```python
from build123d import *

# Parameters (mm, degrees)
F0_W     = 25
F0_H     = 25
F1_DEPTH = 17.5
F2_W     = 25
F2_H     = 25
F3_DEPTH = 15


with BuildPart() as f1:
    # F0 (on Front) → F1 (new body)
    with BuildSketch(Plane.XZ):
        with Locations((12.5, 12.5)):
            Rectangle(F0_W, F0_H)
    extrude(amount=F1_DEPTH)

    # F2 (on face) → F3 (join)
    with BuildSketch(Plane.XZ.offset(17.5)):
        Polygon((25, 25), (25, 0), (45, 0), (45, 45), (0, 45), (0, 25), align=None)
        with Locations((12.5, 12.5)):
            Rectangle(F2_W, F2_H)
    extrude(amount=F3_DEPTH)

    # F4: F1 across face


with BuildPart() as f1_1:
    add(f1.part)
    add(f1.part.mirror(Plane(origin=(12.5, 0, 12.5), x_dir=(1, 0, 0), z_dir=(0, 1, 0))))


solid = f1_1.part
```
Work out the finished part from the listing and answer in its coordinate system (mm). A direction names the side the tool comes from. Coordinates: 2 decimals unless noted, no trailing zeros. Loops run counter-clockwise (first coordinate to the right, second up) from the corner with the lowest first, then second, coordinate; pieces in that order, holes last.
1) For faces 1 (the flat face through (27, 17.5, 28)), 2 (the flat face through (12, 0, 25)), 3 (the flat face through (25, 0, 12)), determine the directions among +Z, -Z, +X, -X, +Y, -Y from which every point of the face is accessible in a straight line to the end or side of a thin tool.
Results:
face 1: +Z, +X
face 2: +Z, +X, -X
face 3: +Z, -Z, +X
2) Section D-D (x = 11) is taken. Give the vertices of the cut face in (y, z).
Results:
outline: (-32.5, 0) - (32.5, 0) - (32.5, 45) - (17.5, 45) - (17.5, 25) - (-17.5, 25) - (-17.5, 45) - (-32.5, 45) - close
3) Consider probe 1 along Y at (x, z) = (37, 41.5); probe 2 along Z at (x, y) = (11.5, -12). Determine where each line is inside the solid, lowest interval first.
Results:
probe 1: y = -32.5 to -17.5, 17.5 to 32.5
probe 2: z = 0 to 25
4) Section B-B (x = 33.5) is taken. Give the vertices of the cut face in (y, z).
Results:
outline: (-32.5, 0) - (-17.5, 0) - (-17.5, 45) - (-32.5, 45) - close; (17.5, 0) - (32.5, 0) - (32.5, 45) - (17.5, 45) - close
5) Section A-A (z = 38.5) is taken. Give the vertices of the cut face in (x, y).
Results:
outline: (0, -32.5) - (45, -32.5) - (45, -17.5) - (0, -17.5) - close; (0, 17.5) - (45, 17.5) - (45, 32.5) - (0, 32.5) - close
6) Section C-C (z = 11.5) is taken. Give the vertices of the cut face in (x, y).
Results:
outline: (0, -32.5) - (45, -32.5) - (45, -17.5) - (25, -17.5) - (25, 17.5) - (45, 17.5) - (45, 32.5) - (0, 32.5) - close
7) Flat-ended cylindrical pins translate along their axes: pin 1 (8 mm diameter, centred on y = -11, z = 20, fed in from +X); pin 2 (10 mm diameter, centred on y = -3, z = 34, fed in from -X). Find the tip coordinate at first contact, or state that the pin passes through.
Results:
pin 1: stops at x = 25
pin 2: passes through
